The model under review builds one solid part; all positions refer to its coordinate system, in mm. Coordinates: 2 decimals unless noted, no trailing zeros. Loops run counter-clockwise (first coordinate to the right, second up) from the corner with the lowest first, then second, coordinate; pieces in that order, holes last. Notation, with made-up numbers: M 34,36 L 76,36 A12 cw 76,54 Z; hole C 51.5,-27 d9. An arc over 180 degrees is marked long. Use CSV: the item, a comma, the result in double quotes. Start each with the question number.
1. Add section A-A, the plane y = -64.6. Write out the cut boundary in (x, z), then the cut area to 3 significant figures.
2. For L1, parallel to Y at x = 0, z = 4 (3 decimals); L2, parallel to X at y = -19.5, z = 2.75; L3, parallel to Y at x = 16, z = 3 (3 decimals), list the stretches that pass through material, from the lowest coordinate up.
3. Clearance check with a flat-ended pin moving along its axis: P1, Ø1.5, axis at x = -13.47, y = -78.06, coming from the +Z side. State where the tip first meets the part, or that it passes through.
4. Add section B-B, the plane x = 17. Write out the cut boundary in (y, z) (3 decimals), then the cut area to 3 significant figures.
5. Add section D-D, the plane z = 3.5. State how many separate pieces and enclosed holes the cut face has, then the cut area to 3 significant figures.
6. Add section C-C, the plane y = -17. Write out the cut boundary in (x, z), then the cut area to 3 significant figures.
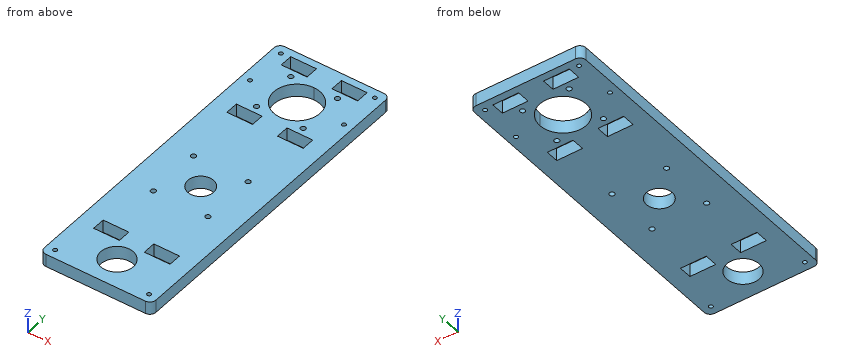
from build123d import *

# Parameters (mm, degrees)
F0_W     = 55
F0_H     = 160
F0_W_2   = 12.7
F0_H_2   = 6.35
F0_R     = 8
F0_R_2   = 6.35
F1_DEPTH = 6.35
F2_D     = 2.5
F3_R     = 3
F4_D     = 2


with BuildPart() as f1:
    # F0 (on Top) → F1 (new body)
    with BuildSketch(Plane.XY):
        with Locations((0, -55)):
            Rectangle(F0_W, F0_H)
        with Locations((-12.5, -107.6)):
            Rectangle(F0_W_2, F0_H_2, mode=Mode.SUBTRACT)
        with Locations((0, -120.735)):
            Circle(F0_R, mode=Mode.SUBTRACT)
        with Locations((12.5, -107.6)):
            Rectangle(F0_W_2, F0_H_2, mode=Mode.SUBTRACT)
        with Locations((0, -64.6)):
            Circle(F0_R_2, mode=Mode.SUBTRACT)
        with Locations((-12.5, -18.25)):
            Rectangle(F0_W_2, F0_H_2, mode=Mode.SUBTRACT)
        with Locations((-12.5, 18.25)):
            Rectangle(F0_W_2, F0_H_2, mode=Mode.SUBTRACT)
        with Locations((12.5, -18.25)):
            Rectangle(F0_W_2, F0_H_2, mode=Mode.SUBTRACT)
        with BuildLine():
            ThreePointArc((0, 11.4), (8.0610173055, 8.0610173055), (11.4, 0))
            ThreePointArc((11.4, 0), (-8.0610173055, -8.0610173055), (0, 11.4))
        make_face(mode=Mode.SUBTRACT)
        with Locations((12.5, 18.25)):
            Rectangle(F0_W_2, F0_H_2, mode=Mode.SUBTRACT)
    extrude(amount=F1_DEPTH)

    # F2 (through all)
    with Locations(Plane(origin=(0, 0, 0), x_dir=(1, 0, 0), z_dir=(0, 0, -1))):
        with Locations((-11.5, -11.5), (11.5, -11.5), (11.5, 11.5), (-11.5, 11.5), (-13.46962, 51.133907857), (13.46962, 51.133907857), (13.46962, 78.057907857), (-13.46962, 78.057907857)):
            Hole(F2_D / 2)

    # F3
    f3_edges = [f1.edges().sort_by_distance(p)[0] for p in [
        (-27.5, -135, 3.175),
        (27.5, -135, 3.175),
        (27.5, 25, 3.175),
        (-27.5, 25, 3.175),
    ]]
    fillet(f3_edges, radius=F3_R)

    # F4 (through all)
    with Locations(Plane(origin=(0, 0, 0), x_dir=(1, 0, 0), z_dir=(0, 0, -1))):
        with Locations((-23.175, 130.675), (23.175, 130.675), (23.175, 0), (23.175, -20.675), (-23.175, -20.675), (-23.175, 0)):
            Hole(F4_D / 2)


solid = f1.part
Computed:
1,outline,"M -27.5,0 L -6.35,0 L -6.35,6.35 L -27.5,6.35 Z; M 6.35,0 L 27.5,0 L 27.5,6.35 L 6.35,6.35 Z"
1,area,"269 mm^2"
2,L1,"y = -135 to -128.735, -112.735 to -70.95, -58.25 to -11.4, 11.4 to 25"
2,L2,"x = -27.5 to -18.85, -6.15 to 6.15, 18.85 to 27.5"
2,L3,"y = -135 to -110.775, -104.425 to -21.425, -15.075 to 15.075, 21.425 to 25"
3,P1,"passes through"
4,outline,"M -135,0 L -110.775,0 L -110.775,6.35 L -135,6.35 Z; M -104.425,0 L -21.425,0 L -21.425,6.35 L -104.425,6.35 Z; M -15.075,0 L 15.075,0 L 15.075,6.35 L -15.075,6.35 Z; M 21.425,0 L 25,0 L 25,6.35 L 21.425,6.35 Z"
4,area,"895 mm^2"
5,separate pieces,"1"
5,enclosed holes,"23"
5,area,"7,510 mm^2"
6,outline,"M -27.5,0 L -18.85,0 L -18.85,6.35 L -27.5,6.35 Z; M -6.15,0 L 6.15,0 L 6.15,6.35 L -6.15,6.35 Z; M 18.85,0 L 27.5,0 L 27.5,6.35 L 18.85,6.35 Z"
6,area,"188 mm^2"
